Build history of the part. All positions in model axes, mm. Round coordinates to 2 decimals unless told otherwise and drop trailing zeros. Write each loop counter-clockwise with the first axis right and the second up, starting at its lowest first coordinate (ties: lowest second). Pieces come first, ordered by that corner, then holes. Notation, with made-up numbers: (76, 72.5) -> (131, 72.5) arc R15 cw to (131, 80.5) -> close; hole circle Ø3 at (25, 48.5). An arc over 180 degrees is marked (long way). Return JSON: item names as keys, results as strings.
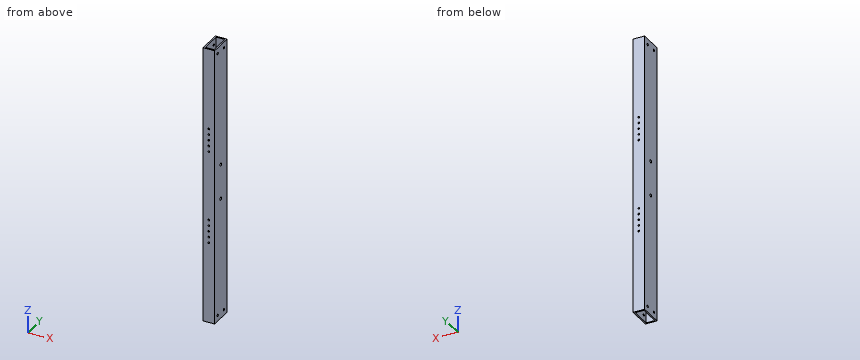
from build123d import *

# Parameters (mm, degrees)
SKETCH1_W               = 25.4
SKETCH1_H               = 50.8
SKETCH1_W_2             = 19.05
SKETCH1_H_2             = 44.45
BOSS_EXTRUDE1_DEPTH     = 304.8
F_10_CLEARANCE_HOLE1_D  = 5.1054
F_1_4_CLEARANCE_HOLE2_D = 6.7564
SKETCH7_R               = 1.905
CUT_EXTRUDE1_DEPTH      = 310.265209812


with BuildPart() as part:
    # Sketch1 → Boss-Extrude1 (new, symmetric)
    with BuildSketch(Plane.XY):
        Rectangle(SKETCH1_W, SKETCH1_H)
        Rectangle(SKETCH1_W_2, SKETCH1_H_2, mode=Mode.SUBTRACT)
    extrude(amount=BOSS_EXTRUDE1_DEPTH, both=True)

    # #10 Clearance Hole1 (through all)
    with Locations(Plane(origin=(12.7, 0, 0), x_dir=(0, 0, -1), z_dir=(1, 0, 0))):
        with Locations((-292.1, 12.7), (-292.1, -12.7)):
            f_10_clearance_hole1 = Hole(F_10_CLEARANCE_HOLE1_D / 2)

    # Mirror1: #10 Clearance Hole1 across plane
    add(f_10_clearance_hole1.mirror(Plane.XY), mode=Mode.SUBTRACT)

    # 1/4 Clearance Hole2 (through all)
    with Locations(Plane(origin=(12.7, 0, 0), x_dir=(0, 0, -1), z_dir=(1, 0, 0))):
        with Locations((-38.1, 0), (38.1, 0)):
            Hole(F_1_4_CLEARANCE_HOLE2_D / 2)

    # Sketch7 → Cut-Extrude1 (cut, through all)
    with BuildSketch(Plane(origin=(0, 25.4, 0), x_dir=(1, 0, 0), z_dir=(0, 1, 0))):
        with Locations(Location((0, 127, 0), (0, 0, 270))):
            Circle(SKETCH7_R)
        with Locations(Location((0, 114.3, 0), (0, 0, 270))):
            Circle(SKETCH7_R)
        with Locations(Location((0, 101.6, 0), (0, 0, 270))):
            Circle(SKETCH7_R)
        with Locations(Location((0, 88.9, 0), (0, 0, 270))):
            Circle(SKETCH7_R)
        with Locations(Location((0, 76.2, 0), (0, 0, 270))):
            Circle(SKETCH7_R)
    cut_extrude1 = extrude(amount=-CUT_EXTRUDE1_DEPTH, mode=Mode.SUBTRACT)

    # Mirror2: Cut-Extrude1 across plane
    add(cut_extrude1.mirror(Plane.XY), mode=Mode.SUBTRACT)


solid = part.part
Q1. Pin check, flat tip, straight feed: pin 1 Ø3.5 at (x, z) = (0, -127) entering from +Y. Stop position of the tip, or through.
Verdict:
{"pin 1": "passes through"}
Q2. Saw through at A-A on z = -184.5. List the corners of the cut face in (x, y) (3 decimals).
Verdict:
{"outline": "(-12.7, -25.4) -> (12.7, -25.4) -> (12.7, 25.4) -> (-12.7, 25.4) -> close; hole (-9.525, -22.225) -> (9.525, -22.225) -> (9.525, 22.225) -> (-9.525, 22.225) -> close"}
Q3. Wall check: L1, parallel to Y at x = 11.6, z = 292.1; L2, parallel to Y at x = 1.5, z = 171.5 (3 decimals); L3, parallel to X at y = 19, z = 55 (3 decimals). Give the ranges that are in metal, low to high.
Verdict:
{"L1": "y = -25.4 to -15.25, -10.15 to 10.15, 15.25 to 25.4", "L2": "y = -25.4 to -22.225, 22.225 to 25.4", "L3": "x = -12.7 to -9.525, 9.525 to 12.7"}
